Design review of the part built by this model. Coordinates are the model's own, in mm. Give positions to 0.01 mm unless a question says otherwise; leave off trailing zeros. Order: outer loops, then holes, each group sorted by start corner. A loop starts at its lowest first (then second) coordinate and runs counter-clockwise, first axis right, second up. Notation, with made-up numbers: M 64,71.5 L 88,71.5 A13 ccw 88,83.5 Z; hole C -27.5,76 d5. An arc over 180 degrees is marked long. Answer as a JSON object with one key per item and string values.
Autodesk Inventor part; units mm, degrees
ref_plane "YZ Plane" through (0, 0, 0) normal (1, 0, 0) x (0, 1, 0)
ref_plane "XZ Plane" through (0, 0, 0) normal (0, 1, 0) x (-1, 0, 0)
ref_plane "XY Plane" through (0, 0, 0) normal (0, 0, 1) x (1, 0, 0)
sketch "Эскиз1" plane through (0, 0, 0) normal (0, 0, 1) x (1, 0, 0)
  circle A0 centre (0, 0) radius 55
  circle A1 centre (0, 0) radius 24
  line L0 (0, -55) -> (0, 55)
  point P0 (0, 24)
  point P1 (0, -24)
  dimension "d0" = 110
  dimension "d1" = 48
revolve "Вращение1" add sketch "Эскиз1" angle 360 about axis through (0, -55, 0) along (0, 1, 0) picked at (-44.4519, -0.9643) contours L0 A1 A0
sketch "Эскиз2" plane through (0, 0, 0) normal (0, 0, 1) x (1, 0, 0)
  line L0 (15, 0) -> (-15, 0)
  line L1 (-15, 0) -> (-15, 40)
  line L2 (-15, 40) -> (15, 40)
  line L3 (15, 40) -> (15, 0)
  line L4 (-40, 0) -> (40, 0)
  line L5 (40, 0) -> (40, -20)
  line L6 (40, -20) -> (-40, -20)
  line L7 (-40, -20) -> (-40, 0)
  point P0 (0, 0)
  point P1 (0, 0)
  point P2 (0, 0)
  point P3 (0, 0)
  dimension "d3" = 0
  dimension "d4" = 0
  dimension "d5" = 80
  dimension "d6" = 20
  dimension "d7" = 30
  dimension "d8" = 60
extrude "Выдавливание1" cut sketch "Эскиз2" against normal mid plane 1000
properties part number "1_2"
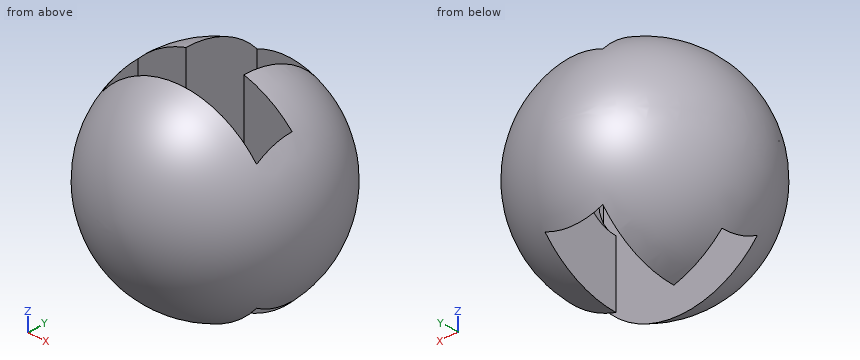
(1) We need section D-D (x = -44). Write out the cut boundary in (y, z).
Checked values:
{"outline": "C 0,0 d66"}
(2) We need section B-B (z = 3.5). Write out the cut boundary in (x, y), plus the area to 3 significant figures.
Checked values:
{"outline": "C 0,0 d109.78; hole M -40,-20 L -12.8,-20 A23.74 ccw 12.8,-20 L 40,-20 L 40,0 L 23.74,0 A23.74 ccw 15,18.41 L 15,40 L -15,40 L -15,18.41 A23.74 ccw -23.74,0 L -40,0 Z", "area": "6,380 mm^2"}
(3) We need section C-C (x = 5). Write out the cut boundary in (y, z), plus the area to 3 significant figures.
Checked values:
{"outline": "M -20,-50.99 L -20,-12.29 A23.47 cw -20,12.29 L -20,50.99 A54.77 ccw Z; M 40,-37.42 A54.77 ccw 40,37.42 Z", "area": "3,270 mm^2"}
(4) To check wall thickness, follow L1, parallel to X at y = 25, z = 40; L2, parallel to Y at x = -1, z = -27.5; L3, parallel to Y at x = 18, z = -33.5. State the ranges of each line that lie inside material, in increasing order. Write a range as from..to.
Checked values:
{"L1": "x = -28.28..-15, 15..28.28", "L2": "y = -47.62..-20, 40..47.62", "L3": "y = -39.73..-20, 0..39.73"}
(5) We need section A-A (y = 11.5). Write out the cut boundary in (x, z), plus the area to 3 significant figures.
Checked values:
{"outline": "M -15,-51.65 L -15,-14.79 A21.07 cw -15,14.79 L -15,51.65 A53.78 ccw Z; M 15,-51.65 A53.78 ccw 15,51.65 L 15,14.79 A21.07 cw 15,-14.79 Z", "area": "5,660 mm^2"}
(6) Insertion check: pin 1 (5 mm diameter, centred on x = 22, y = 18, fed in from +Z); pin 2 (5 mm diameter, centred on x = -9.5, z = -28, fed in from -Y); pin 3 (5 mm diameter, centred on y = 35, z = 9.5, fed in from +X). Each pin has a flat end and moves straight along its axis. Give the tip position at first contact, or say it passes through.
Checked values:
{"pin 1": "stops at z = 48.51", "pin 2": "stops at y = -47.88", "pin 3": "stops at x = 43.41"}
